Can you work these out from the drawing? Everything is in mm from the part's minimum corner. A direction names the side the tool comes from. Coordinates: 2 decimals unless noted, no trailing zeros. Order: outer loops, then holes, each group sorted by start corner. A loop starts at its lowest first (then second) coordinate and runs counter-clockwise, first axis right, second up. Notation, with made-up numbers: (-4, -26) -> (55, -26) arc R31 cw to (55, 10) -> close; hole circle Ø4 at (-33, 9.25). An arc over 180 degrees is marked (long way). Use a Markdown table: item, result. Add a question column.
1) If we section it at A-A (z = 36): Write out the boundary of the cut face in (x, y).
2) Which directions (+Z, -Z, +X, -X, +Y, -Y) give clear straight access to the entire face, cutting with the end or side of a thin tool? Please do the marked faces 4, 5 and 6.
3) Will these pins go through, and if not, where does the flat tip stop? pin 1 Ø4 at (x, z) = (36, 3) entering from +Y; pin 2 Ø8 at (x, y) = (36.5, 27.5) entering from -Z.
4) If we section it at D-D (z = 21): Write out the boundary of the cut face in (x, y), plus the area to 3 significant figures.
5) If we section it at B-B (x = 25): Write out the boundary of the cut face in (y, z), plus the area to 4 significant figures.
6) If I drill on L1, parallel to Y at x = 27.5, z = 29; L2, parallel to Y at x = 25, z = 3; L3, parallel to Z at x = 8, y = 12.75, over which ranges is the centre line in solid material (lowest first)? Write a range as [from, to].
7) Thinking about a two-plate mould opening in Y: for the marked faces 1, 2 and 3, which applies, +Y half, -Y half, draft (parallel to the pull), parting line (faces both ways), or undercut?
8) If we section it at C-C (y = 15.38): Write out the boundary of the cut face in (x, z), plus the area to 3 significant figures.
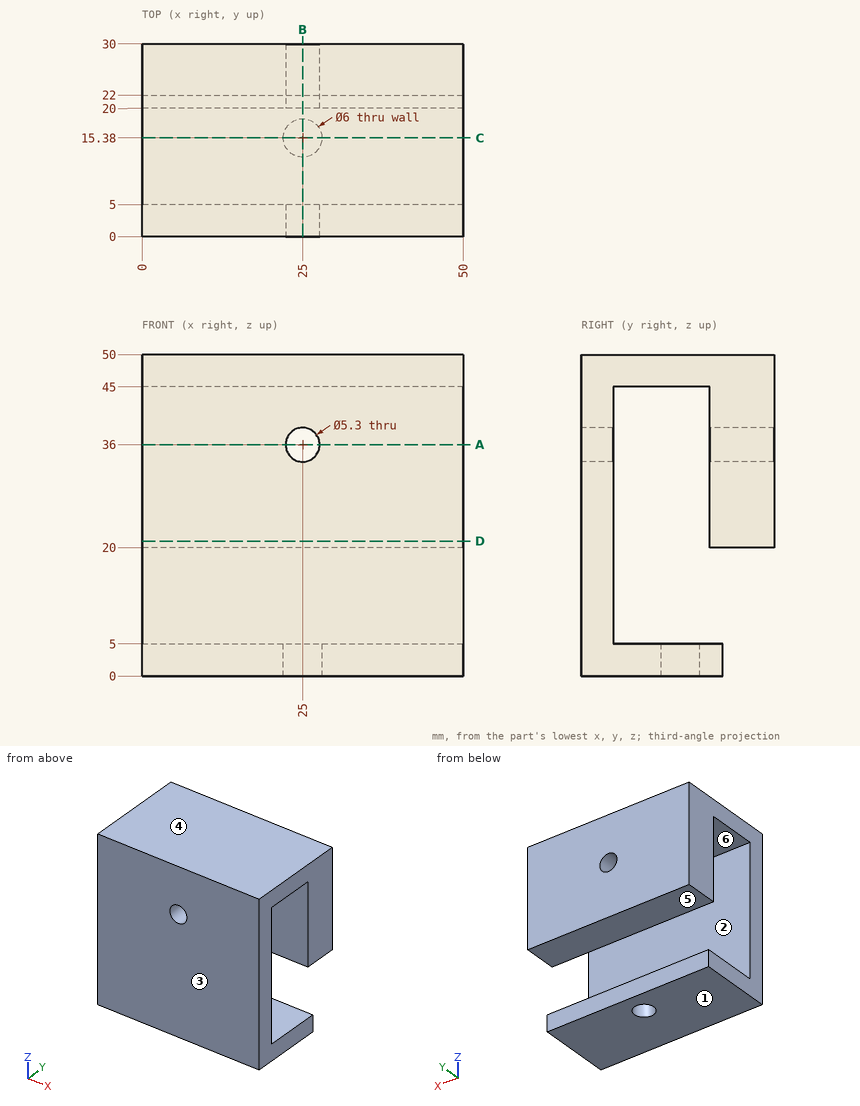
Answer sheet:
| question | item | result |
|---|---|---|
| 1 | outline | (0, 0) -> (22.35, 0) -> (22.35, 5) -> (0, 5) -> close; (0, 20) -> (22.35, 20) -> (22.35, 30) -> (0, 30) -> close; (27.65, 0) -> (50, 0) -> (50, 5) -> (27.65, 5) -> close; (27.65, 20) -> (50, 20) -> (50, 30) -> (27.65, 30) -> close |
| 2 | face 4 | +Z, +X, -X, +Y, -Y |
| 2 | face 5 | +X, -X, +Y |
| 2 | face 6 | +X, -X |
| 3 | pin 1 | y = 22 |
| 3 | pin 2 | z = 20 |
| 4 | outline | (0, 0) -> (50, 0) -> (50, 5) -> (0, 5) -> close; (0, 20) -> (50, 20) -> (50, 30) -> (0, 30) -> close |
| 4 | area | 750 mm2 |
| 5 | outline | (0, 0) -> (12.38, 0) -> (12.38, 5) -> (5, 5) -> (5, 33.35) -> (0, 33.35) -> close; (0, 38.65) -> (5, 38.65) -> (5, 45) -> (20, 45) -> (20, 38.65) -> (30, 38.65) -> (30, 50) -> (0, 50) -> close; (18.38, 0) -> (22, 0) -> (22, 5) -> (18.38, 5) -> close; (20, 20) -> (30, 20) -> (30, 33.35) -> (20, 33.35) -> close |
| 5 | area | 600.5 mm2 |
| 6 | L1 | [0, 5], [20, 30] |
| 6 | L2 | [0, 12.38], [18.38, 22] |
| 6 | L3 | [0, 5], [45, 50] |
| 7 | face 1 | draft |
| 7 | face 2 | undercut |
| 7 | face 3 | -Y half |
| 8 | outline | (0, 0) -> (22, 0) -> (22, 5) -> (0, 5) -> close; (0, 45) -> (50, 45) -> (50, 50) -> (0, 50) -> close; (28, 0) -> (50, 0) -> (50, 5) -> (28, 5) -> close |
| 8 | area | 470 mm2 |
